```python
from build123d import *

# Parameters (mm, degrees)
SKETCH1_W           = 139.7
SKETCH1_H           = 203.2
BOSS_EXTRUDE1_DEPTH = 10.16
SKETCH2_W           = 38.1
SKETCH2_H           = 50.8
BOSS_EXTRUDE2_DEPTH = 76.2
CUT_EXTRUDE1_DEPTH  = 89.9
SKETCH4_W           = 38.1
SKETCH4_H           = 19.05
BOSS_EXTRUDE3_DEPTH = 25.4
BOSS_EXTRUDE4_DEPTH = 38.1
CUT_EXTRUDE2_DEPTH  = 82.219688091
SKETCH7_W           = 38.1
SKETCH7_H           = 12.7
BOSS_EXTRUDE5_DEPTH = 317.5
FILLET1_R           = 2.54
FILLET2_R           = 19.05


with BuildPart() as part:
    # Sketch1 → Boss-Extrude1 (new body)
    with BuildSketch(Plane(origin=(0, 0, 0), x_dir=(1, 0, 0), z_dir=(0, 1, 0))):
        Rectangle(SKETCH1_W, SKETCH1_H)
    extrude(amount=BOSS_EXTRUDE1_DEPTH)

    # Sketch2 → Boss-Extrude2 (add)
    with BuildSketch(Plane(origin=(0, 10.16, 0), x_dir=(1, 0, 0), z_dir=(0, 1, 0))):
        with Locations((0, 63.5)):
            Rectangle(SKETCH2_W, SKETCH2_H)
    extrude(amount=BOSS_EXTRUDE2_DEPTH)

    # Sketch3 → Cut-Extrude1 (cut, through all)
    with BuildSketch(Plane.ZY.offset(19.05)):
        Polygon((-38.1, 10.16), (-38.1, 22.86), (-55.138837989, 14.340581006), (-55.138837989, 10.16), align=None)
        Polygon((-38.1, 86.36), (-69.85, 86.36), (-38.1, 22.86), align=None)
    extrude(amount=-CUT_EXTRUDE1_DEPTH, mode=Mode.SUBTRACT)

    # Sketch4 → Boss-Extrude3 (add)
    with BuildSketch(Plane(origin=(0, 86.36, 0), x_dir=(1, 0, 0), z_dir=(0, 1, 0))):
        with Locations((0, 79.375)):
            Rectangle(SKETCH4_W, SKETCH4_H)
    extrude(amount=BOSS_EXTRUDE3_DEPTH)

    # Sketch5 → Boss-Extrude4 (add)
    with BuildSketch(Plane.ZY.offset(19.05)):
        Polygon((-88.9, 111.76), (-38.177367303, 399.422344655), (-19.701795091, 396.16460279), (-69.85, 111.76), align=None)
    extrude(amount=-BOSS_EXTRUDE4_DEPTH)

    # Sketch6 → Cut-Extrude2 (cut, through all)
    with BuildSketch(Plane(origin=(0, 15.315029856, -86.85585039), x_dir=(1, 0, 0), z_dir=(0, -0.173648178, 0.984807753))):
        with BuildLine():
            Line((6.35, 356.628790374), (6.35, 128.028790374))
            ThreePointArc((6.35, 128.028790374), (0, 121.678790374), (-6.35, 128.028790374))
            Line((-6.35, 128.028790374), (-6.35, 356.628790374))
            ThreePointArc((-6.35, 356.628790374), (0, 362.978790374), (6.35, 356.628790374))
        make_face()
    extrude(amount=-CUT_EXTRUDE2_DEPTH, mode=Mode.SUBTRACT)

    # Sketch7 → Boss-Extrude5 (add)
    with BuildSketch(Plane(origin=(0, 18.572771721, -105.331422603), x_dir=(1, 0, 0), z_dir=(0, -0.173648178, 0.984807753))):
        with Locations((0, 393.074791482)):
            Rectangle(SKETCH7_W, SKETCH7_H)
    extrude(amount=BOSS_EXTRUDE5_DEPTH)

    # Fillet1
    fillet1_edges = [part.edges().sort_by_distance(p)[0] for p in [
        (-19.05, 384.362754913, 120.366195344),
        (-19.05, 370.226825518, 127.398649594),
        (19.05, 370.226825518, 127.398649594),
        (0, 411.929403118, -35.972035447),
        (19.05, 384.362754913, 120.366195344),
        (-19.05, 350.542577477, 275.601760206),
        (0, 344.289048246, 274.499094278),
        (19.05, 350.542577477, 275.601760206),
        (0, 356.796106709, 276.704426134),
        (0, 10.16, -88.9),
        (19.05, 60.96, -88.9),
        (-19.05, 10.16, -72.019418994),
        (-19.05, 60.96, -88.9),
        (0, 22.86, -38.1),
        (19.05, 10.16, -72.019418994),
        (19.05, 12.250290503, -55.138837989),
        (0, 10.16, -55.138837989),
        (19.05, 18.600290503, -46.619418994),
        (-19.05, 18.600290503, -46.619418994),
        (-19.05, 12.250290503, -55.138837989),
        (19.05, 54.61, -53.975),
        (-19.05, 54.61, -53.975),
        (-19.05, 99.06, -69.85),
        (19.05, 99.06, -69.85),
        (0, 111.76, -88.9),
        (-19.05, 253.962301395, -44.775897545),
        (-19.05, 261.844701559, -62.436017724),
        (19.05, 261.844701559, -62.436017724),
        (19.05, 253.962301395, -44.775897545),
        (0, 376.037098661, -42.300817123),
        (6.35, 257.22004326, -63.251469758),
        (0, 138.402987859, -84.202122394),
        (-6.35, 257.22004326, -63.251469758),
        (0, 372.779356796, -23.82524491),
        (-6.35, 253.962301395, -44.775897545),
        (0, 135.145245994, -65.726550181),
        (6.35, 253.962301395, -44.775897545),
    ]]
    fillet(fillet1_edges, radius=FILLET1_R)

    # Fillet2
    fillet2_edges = [part.edges().sort_by_distance(p)[0] for p in [
        (69.85, 5.08, 101.6),
        (-69.85, 5.08, 101.6),
        (-69.85, 5.08, -101.6),
        (69.85, 5.08, -101.6),
    ]]
    fillet(fillet2_edges, radius=FILLET2_R)


solid = part.part
```
Read the model definition and answer for the solid it produces. Units are mm, in the model's axes. A direction names the side the tool comes from. Give positions to 0.01 mm unless a question says otherwise; leave off trailing zeros. Write each loop counter-clockwise with the first axis right and the second up, starting at its lowest first coordinate (ties: lowest second). Pieces come first, ordered by that corner, then holes. Notation, with made-up numbers: (-25, -10.75) - (20, -10.75) arc R18 ccw to (20, 10.25) - close; hole circle Ø7 at (52.5, 18.5). An arc over 180 degrees is marked (long way). Write item = value, one per line. Start each with the question number.
Item 1: Find section B-B (x = -56.5). Give the vertices of the cut face in (y, z), then the cut area to 3 significant figures.
Item 2: Find the intervals of material crossed by probe 1 along X at (y, z) = (78, -85); probe 2 along Y at (x, z) = (-21, 56); probe 3 along Z at (x, y) = (-17, 144.5), in increasing order. Write a range as [from, to].
Item 3: Each of these flat-tipped pins is pushed along its axis until it touches: P1, Ø16, axis at y = 214, z = -53.5, coming from the +X side; P2, Ø4, axis at x = -1.5, z = 74, coming from the +Y side; P3, Ø3, axis at x = -2, y = 358.5, coming from the +Z side. Where does it stop, or does it pass through?
Item 4: A tool of negligible diameter and unlimited length cuts with its end or side. For faces 1 (the flat face through (-0.231, 18.084, -47.652)), 2 (the flat face through (-1, 5, 101.6)), 3 (the cylindrical face through (-18.326, 55.24, -55.144)), from which of +Z, -Z, +X, -X, +Y, -Y can it reach the whole face along a straight path? Write none if from no direction.
Item 5: Find section A-A (x = -32). Give the vertices of the cut face in (y, z).
Item 6: The mould has two halves that part along Y. Classify faces 4 (the cylindrical face through (18.286, 253.219, -45.642)), 5 (the cylindrical face through (0.14, 136.76, -74.87)), 6 (the flat face through (-1, 5, -101.6)): +Y half, -Y half, draft (parallel to the pull), parting line (faces both ways), or undercut.
Response:
q1.outline = (0, -100.73) - (10.16, -100.73) - (10.16, 100.73) - (0, 100.73) - close
q1.area = 2,050 mm²
q2.probe_1 = [-19.05, 19.05]
q2.probe_2 = [0, 10.16]
q2.probe_3 = [-83.08, -64.13]
q3.P1 = 19.05
q3.P2 = 392.89
q3.P3 = 274.91
q4.face_1 = +Z, +X, -X
q4.face_2 = +Z, +X, -X, -Y
q4.face_3 = +Z, -X
q5.outline = (0, -101.6) - (10.16, -101.6) - (10.16, 101.6) - (0, 101.6) - close
q6.face_4 = undercut
q6.face_5 = +Y half
q6.face_6 = draft
